from build123d import *

# Parameters (mm, degrees)
F0_R     = 100
F1_DEPTH = 500
F3_DEPTH = 300


# Not quite as in the source:
# - ends of sketch curves that miss each other by under 0.0002 mm in the source are joined


with BuildPart() as f1:
    # F0 (on Top) → F1 (new body)
    with BuildSketch(Plane.XY):
        with BuildLine():
            Line((344.892811266, 199.9347809243), (-349.9812287722, 199.9999991191))
            ThreePointArc((-349.9812287722, 199.9999991191), (-550, 0), (-349.9812287722, -199.9999991191))
            Line((-349.9812287722, -199.9999991191), (344.892811266, -199.9347809243))
            Line((344.892811266, -199.9347809243), (355.1449138709, -199.9338187015))
            ThreePointArc((355.1449138709, -199.9338187015), (550, 9.74749e-05), (355.1447188571, 199.9338187198))
            Line((355.1447188571, 199.9338187198), (344.892811266, 199.9347809243))
        make_face()
        with Locations((-350, 0)):
            Circle(F0_R, mode=Mode.SUBTRACT)
        with Locations((350, 0)):
            Circle(F0_R, mode=Mode.SUBTRACT)
    extrude(amount=F1_DEPTH)


with BuildPart() as f3:
    # F2 (on Front) → F3 (new body, symmetric)
    with BuildSketch(Plane.XZ):
        with BuildLine():
            Line((-550, 100), (-550, 0))
            Line((-550, 0), (-150, 0))
            ThreePointArc((-150, 0), (-114.6446609407, 14.6446609407), (-100, 50))
            Line((-100, 50), (-100, 150))
            ThreePointArc((-100, 150), (-85.3553390593, 185.3553390593), (-50, 200))
            Line((-50, 200), (150, 200))
            ThreePointArc((150, 200), (185.3553390593, 214.6446609407), (200, 250))
            Line((200, 250), (200, 350))
            ThreePointArc((200, 350), (214.6446609407, 385.3553390593), (250, 400))
            Line((250, 400), (550, 400))
            Line((550, 400), (550, 500))
            Line((550, 500), (150, 500))
            ThreePointArc((150, 500), (114.6446609407, 485.3553390593), (100, 450))
            Line((100, 450), (100, 350))
            ThreePointArc((100, 350), (85.3553390593, 314.6446609407), (50, 300))
            Line((50, 300), (-150, 300))
            ThreePointArc((-150, 300), (-185.3553390593, 285.3553390593), (-200, 250))
            Line((-200, 250), (-200, 150))
            ThreePointArc((-200, 150), (-214.6446609407, 114.6446609407), (-250, 100))
            Line((-250, 100), (-550, 100))
        make_face()
    extrude(amount=F3_DEPTH, both=True)


with BuildPart() as f1_1:
    add(f1.part)

    # F4: intersect F3
    add(f3.part, mode=Mode.INTERSECT)


solid = f1_1.part
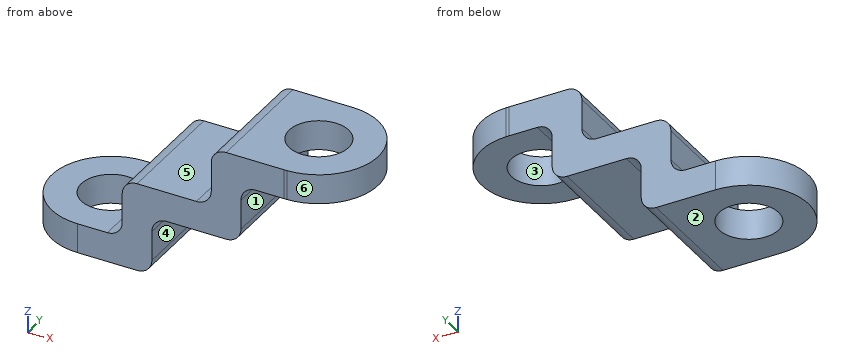
For this review, take the finished solid that the model builds, in its own axes (mm). Face numbers are marked on the shaded views. A direction names the side the tool comes from. Round coordinates to 2 decimals unless told otherwise and drop trailing zeros. Loops run counter-clockwise (first coordinate to the right, second up) from the corner with the lowest first, then second, coordinate; pieces in that order, holes last. Notation, with made-up numbers: (-13, 33) - (43, 33) arc R23 ccw to (43, 63) - close; hole circle Ø6 at (-39, 40.5). An arc over 180 degrees is marked (long way). Use one line per item in the form item = value.
1) Tool access review of the marked faces 4, 5 and 6: name each direction out of +Z, -Z, +X, -X, +Y, -Y from which nothing blocks a thin tool from reaching the whole face with its end or side.
Solutions:
face_4 = -Z, +X, +Y, -Y
face_5 = +Z, -X, +Y, -Y
face_6 = +Z, -Z, +X
2) We need section D-D on x = -87.5. Write out the cut boundary in (y, z), then the cut area to 3 significant figures.
Solutions:
outline = (-199.98, 183.07) - (199.98, 183.07) - (199.98, 300) - (-199.98, 300) - close
area = 46,800 mm2
3) Wall thickness on probe 1 along Y at (x, z) = (-350, 35.5); probe 2 along X at (y, z) = (0, 426.5); probe 3 along Y at (x, z) = (350, 476): over which ranges is each line inside the solid? List them lowest first.
Solutions:
probe_1 = -200 to -100, 100 to 200
probe_2 = 100 to 250, 450 to 550
probe_3 = -199.93 to -100, 100 to 199.93
4) Mouldability with a two-part tool opening along X and no side actions: class the marked faces 1, 2 and 3 as pulls with the +X half, pulls with the -X half, needs draft (parallel to the pull), parting line crosses it, or undercut.
Solutions:
face_1 = pulls with the +X half
face_2 = needs draft
face_3 = undercut
5) Clearance check with flat-ended pins moving along their axes: P1, Ø1, axis at x = 71, y = -97.5, coming from the +Z side; P2, Ø6, axis at x = 25, y = 1.5, coming from the -Z side; P3, Ø10, axis at x = 88, z = 217.5, coming from the +Y side. State where each tip first meets the part, or that it passes through.
Solutions:
P1 = 304.86
P2 = 200
P3 = 199.96
6) We need section B-B on z = 68. Write out the cut boundary in (x, y).
Solutions:
outline = (-349.98, -200) - (-100, -199.98) - (-100, 199.98) - (-349.98, 200) arc R200 ccw to start; hole circle Ø200 at (-350, 0)
7) We need section C-C on y = -124. Write out the cut boundary in (x, z).
Solutions:
outline = (-506.92, 0) - (-150, 0) arc R50 ccw to (-100, 50) - (-100, 150) arc R50 cw to (-50, 200) - (150, 200) arc R50 ccw to (200, 250) - (200, 350) arc R50 cw to (250, 400) - (506.92, 400) - (506.92, 500) - (150, 500) arc R50 ccw to (100, 450) - (100, 350) arc R50 cw to (50, 300) - (-150, 300) arc R50 ccw to (-200, 250) - (-200, 150) arc R50 cw to (-250, 100) - (-506.92, 100) - close
8) We need section A-A on y = 73. Write out the cut boundary in (x, z).
Solutions:
outline = (-536.2, 0) - (-418.34, 0) - (-418.34, 100) - (-536.2, 100) - close; (-281.66, 0) - (-150, 0) arc R50 ccw to (-100, 50) - (-100, 150) arc R50 cw to (-50, 200) - (150, 200) arc R50 ccw to (200, 250) - (200, 350) arc R50 cw to (250, 400) - (281.66, 400) - (281.66, 500) - (150, 500) arc R50 ccw to (100, 450) - (100, 350) arc R50 cw to (50, 300) - (-150, 300) arc R50 ccw to (-200, 250) - (-200, 150) arc R50 cw to (-250, 100) - (-281.66, 100) - close; (418.34, 400) - (536.2, 400) - (536.2, 500) - (418.34, 500) - close
